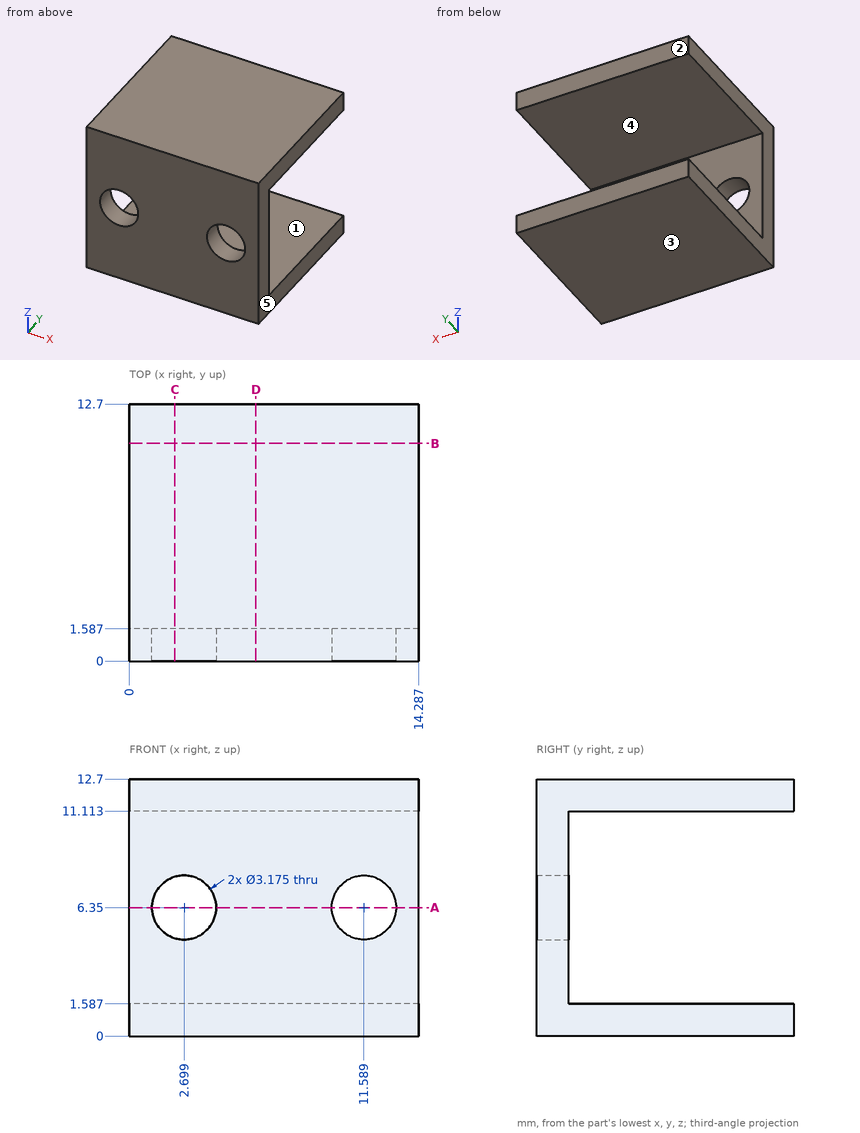
Study the drawing (mm; zero at the part's minimum x, y, z) and answer. A direction names the side the tool comes from. Give positions to 0.01 mm unless a question says otherwise; leave off trailing zeros. Order: outer loops, then holes, each group sorted by start corner. A loop starts at its lowest first (then second) coordinate and runs counter-clockwise, first axis right, second up.
1) Determine the mould class of the marked faces 1, 2 and 3 for opening direction Z: pulls with the +Z half, pulls with the -Z half, needs draft (parallel to the pull), parting line crosses it, or undercut.
Reported:
face 1: undercut
face 2: needs draft
face 3: pulls with the -Z half
2) Given P1, Ø2.5, axis at x = 2.7, z = 6.35, coming from the +Y side; P2, Ø4, axis at x = 11.59, z = 6.35, coming from the +Y side, each flat-ended and moving along its own axis, determine where each tip first touches the part or whether it passes through.
Reported:
P1: passes through
P2: stops at y = 1.59
3) For the marked faces 4 and 5, determine the directions among +Z, -Z, +X, -X, +Y, -Y from which every point of the face is accessible in a straight line to the end or side of a thin tool.
Reported:
face 4: +X, -X, +Y
face 5: +Z, -Z, +X, +Y, -Y
4) Find section B-B on y = 10.75. Write down the section's boundary in (x, z).
Reported:
outline: (0, 0) - (14.29, 0) - (14.29, 1.59) - (0, 1.59) - close; (0, 11.11) - (14.29, 11.11) - (14.29, 12.7) - (0, 12.7) - close
5) Consider line 1 along Z through (x, y) = (4, 4); line 2 along Y through (x, z) = (7.5, 9.5); line 3 along Z through (x, y) = (3.5, 0.75). Determine where each line is inside the solid, lowest interval first.
Reported:
line 1: z = 0 to 1.59, 11.11 to 12.7
line 2: y = 0 to 1.59
line 3: z = 0 to 4.98, 7.72 to 12.7
6) Find section D-D on x = 6.25. Write down the section's boundary in (y, z).
Reported:
outline: (0, 0) - (12.7, 0) - (12.7, 1.59) - (1.59, 1.59) - (1.59, 11.11) - (12.7, 11.11) - (12.7, 12.7) - (0, 12.7) - close
7) Find section A-A on z = 6.35. Write down the section's boundary in (x, y).
Reported:
outline: (0, 0) - (1.11, 0) - (1.11, 1.59) - (0, 1.59) - close; (4.29, 0) - (10, 0) - (10, 1.59) - (4.29, 1.59) - close; (13.18, 0) - (14.29, 0) - (14.29, 1.59) - (13.18, 1.59) - close
8) Find section C-C on x = 2.25. Write down the section's boundary in (y, z).
Reported:
outline: (0, 0) - (12.7, 0) - (12.7, 1.59) - (1.59, 1.59) - (1.59, 4.83) - (0, 4.83) - close; (0, 7.87) - (1.59, 7.87) - (1.59, 11.11) - (12.7, 11.11) - (12.7, 12.7) - (0, 12.7) - close
